Autodesk Inventor part; units mm, degrees
ref_plane "YZ Plane" through (0, 0, 0) normal (1, 0, 0) x (0, 1, 0)
ref_plane "XZ Plane" through (0, 0, 0) normal (0, 1, 0) x (-1, 0, 0)
ref_plane "XY Plane" through (0, 0, 0) normal (0, 0, 1) x (1, 0, 0)
sketch "Sketch1" plane through (0, 0, 0) normal (1, 0, 0) x (0, 1, 0)
  point P0 (0, 0)
sketch "Sketch2" plane through (0, 0, 0) normal (1, 0, 0) x (0, 1, 0)
  line L0 (25.8289, -95.4545) -> (-24.1711, -95.4545)
  line L1 (-24.1711, -95.4545) -> (-24.1711, 104.5455)
  line L2 (-24.1711, 104.5455) -> (25.8289, 64.5455)
  line L3 (25.8289, 64.5455) -> (25.8289, 24.5455)
  line L4 (25.8289, -95.4545) -> (25.8289, -65.4545)
  line L5 (21.8289, -91.4545) -> (-20.1711, -91.4545)
  line L6 (-20.1711, -91.4545) -> (-20.1711, 24.5455)
  line L7 (21.8289, 62.623) -> (-20.1711, 96.223)
  line L8 (-20.1711, 96.223) -> (-20.1711, 24.5455)
  line L9 (25.8289, 24.5455) -> (21.8289, 24.5455)
  line L10 (25.8289, -65.4545) -> (21.8289, -65.4545)
  line L11 (21.8289, 62.623) -> (21.8289, 24.5455)
  line L12 (21.8289, -65.4545) -> (21.8289, -91.4545)
  point P0 (0, 0)
  dimension "d3" = 200
  dimension "d4" = 40
  dimension "d5" = 50
  dimension "d6" = 30
  dimension "d7" = 40
  dimension "d9" = 51.34
  dimension "d10" = 4
  dimension "d12" = 4
  dimension "d14" = 4
  dimension "d15" = 4
  dimension "d16" = 4
  dimension "d17" = 4
  dimension "d18" = 4
extrude "Extrusion1" add sketch "Sketch2" along normal blind 160
sketch "Sketch3" plane through (0, 25.8289, 64.5455) normal (0, 1, 0) x (1, 0, 0)
  line L0 (1, 1) -> (159, 1)
  line L1 (159, 1) -> (159, 39)
  line L2 (159, 39) -> (1, 39)
  line L3 (1, 39) -> (1, 1)
  line L4 (0, 40) -> (0, 0)
  line L5 (0, 40) -> (160, 40)
  line L6 (0, 0) -> (160, 0)
  line L7 (160, 40) -> (160, 0)
  point P0 (0, 64.5455)
  dimension "d21" = 1
  dimension "d22" = 1
  dimension "d23" = 1
  dimension "d24" = 1
extrude "Extrusion2" add sketch "Sketch3" along normal blind 2 contours L3 L2 L1 L0
sketch "Sketch5" plane through (0, 0, 0) normal (-1, 0, 0) x (0, 0, 1)
  point P0 (0, 0)
sketch "Sketch6" plane through (0, -24.1711, -95.4545) normal (0, -1, 0) x (1, 0, 0)
  circle A0 centre (75, 180) radius 2.5
  circle A1 centre (75, 180) radius 3
  line L0 (0, 200) -> (160, 200)
  line L1 (0, 200) -> (0, 0)
  circle A2 centre (85, 180) radius 2.5
  circle A3 centre (85, 180) radius 3
  circle A4 centre (85, 20) radius 2.5
  circle A5 centre (85, 20) radius 3
  circle A6 centre (75, 20) radius 2.5
  circle A7 centre (75, 20) radius 3
  line L2 (160, 200) -> (160, 0)
  line L3 (0, 0) -> (160, 0)
  point P0 (0, 95.4545)
  dimension "d33" = 5
  dimension "d34" = 6
  dimension "d35" = 20
  dimension "d36" = 75
  dimension "d37" = 5
  dimension "d38" = 6
  dimension "d39" = 5
  dimension "d40" = 6
  dimension "d41" = 5
  dimension "d42" = 6
  dimension "d43" = 75
  dimension "d44" = 20
  dimension "d45" = 20
  dimension "d46" = 20
  dimension "d47" = 75
  dimension "d48" = 75
extrude "Extrusion4" cut sketch "Sketch6" against normal blind 3 contours A1 | A3 | A5 | A7
fillet "Fillet1" radius 2 4 edges at (72.5, -24.1711, -75.4545) (82.5, -24.1711, -75.4545) (72.5, -24.1711, 84.5455) (82.5, -24.1711, 84.5455)
properties part number "Bottom Plastic"
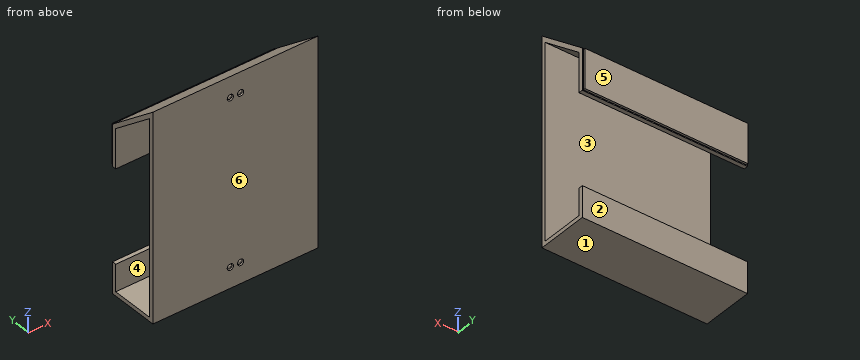
Geometry: final body of the model. Coordinates: model frame, mm. Face numbers are marked on the shaded views. A direction names the side the tool comes from. Coordinates: 2 decimals unless noted, no trailing zeros. Order: outer loops, then holes, each group sorted by start corner. A loop starts at its lowest first (then second) coordinate and runs counter-clockwise, first axis right, second up. Notation, with made-up numbers: (38.5, 36) -> (77.5, 36) arc R18 cw to (77.5, 60) -> close; hole circle Ø4 at (-28, -15). An arc over 180 degrees is marked (long way). Write each question's results on one line, items separated by ' | '. Start each with the question number.
1) Cut plane D-D, the plane z = -17. Output: boundary loops of the cut face in (x, y).
2) Mould query, pull axis Y, two halves, no side actions, for the marked faces 4, 5 and 6. Classes: released by +Y, released by -Y, zero draft, split by the parting line, or undercut.
3) First-contact query: pin 1 (2 mm diameter, centred on x = 74.5, y = 27, fed in from +Z); pin 2 (12 mm diameter, centred on x = 23, y = 6, fed in from +Z); pin 3 (8 mm diameter, centred on x = 73, y = -17, fed in from +Z). Flat tips, straight axial feed; report the tip coordinate or a pass-through.
4) Cut plane A-A, the plane z = 77.5. Output: boundary loops of the cut face in (x, y), and give its area (3 significant figures).
5) Cut plane B-B, the plane y = 10. Output: boundary loops of the cut face in (x, z), and give its area (3 significant figures).
6) Material intervals for line 1 along Y through (x, z) = (73, 45.5); line 2 along Z through (x, y) = (85, -22.4); line 3 along Y through (x, z) = (10, 22), sorted ascending.
7) Set-up query: the marked faces 1, 2 and 3. Return all of +Z, -Z, +X, -X, +Y, -Y with unobstructed straight access to the full face (end or side cutting, diameter ignored); none if empty.
8) Cut plane C-C, the plane x = 133. Output: boundary loops of the cut face in (y, z), and give its area (3 significant figures).
Checks:
1) outline: (0, -24.17) -> (160, -24.17) -> (160, -20.17) -> (0, -20.17) -> close
2) face 4: undercut | face 5: released by +Y | face 6: released by -Y
3) pin 1: z = 63.55 | pin 2: z = 85.21 | pin 3: z = 102.01
4) outline: (0, -24.17) -> (160, -24.17) -> (160, -20.17) -> (0, -20.17) -> close; (0, 3.23) -> (160, 3.23) -> (160, 9.64) -> (0, 9.64) -> close | area: 1,660 mm^2
5) outline: (0, -95.45) -> (160, -95.45) -> (160, -91.45) -> (0, -91.45) -> close; (0, 72.09) -> (160, 72.09) -> (160, 77.21) -> (0, 77.21) -> close | area: 1,460 mm^2
6) line 1: -24.17 to -20.17, 21.83 to 27.83 | line 2: -95.45 to -78.45, -77.94 to -72.97, -72.45 to 81.55, 82.06 to 87.03, 87.55 to 103.13 | line 3: -24.17 to -20.17
7) face 1: -Z, +X, -X, +Y, -Y | face 2: -Z, +X, -X, +Y | face 3: +X, -X
8) outline: (-24.17, -95.45) -> (25.83, -95.45) -> (25.83, -65.45) -> (21.83, -65.45) -> (21.83, -91.45) -> (-20.17, -91.45) -> (-20.17, 96.22) -> (21.83, 62.62) -> (21.83, 24.55) -> (25.83, 24.55) -> (25.83, 25.55) -> (27.83, 25.55) -> (27.83, 63.55) -> (25.83, 63.55) -> (25.83, 64.55) -> (-24.17, 104.55) -> close | area: 1,540 mm^2
